Model file for the job. Use its own axes, mm. Give positions to 0.01 mm unless a question says otherwise; leave off trailing zeros. Order: outer loops, then holes, each group sorted by start corner. A loop starts at its lowest first (then second) coordinate and runs counter-clockwise, first axis right, second up. Notation, with made-up numbers: (-39, 56.25) - (-9, 56.25) arc R32 cw to (-9, 86.25) - close; hole circle Ø7 at (59.5, -6.5). An arc over 180 degrees is marked (long way). Return JSON: item names as keys, results as strings. Group by question number.
from build123d import *

# Parameters (mm, degrees)
HEX_2_DEPTH   = 60
BORE_SKETCH_W = 62
BORE_SKETCH_H = 1.5


with BuildPart() as part:
    # Hex Sketch → Hex 2 (new body)
    with BuildSketch(Plane(origin=(0, 0, 0), x_dir=(0, 0, -1), z_dir=(1, 0, 0))):
        Polygon((3.175426481, 0), (1.58771324, 2.75), (-1.58771324, 2.75), (-3.175426481, 0), (-1.58771324, -2.75), (1.58771324, -2.75), align=None)
    extrude(amount=HEX_2_DEPTH)

    # Bore Sketch → Bore (revolve, cut)
    with BuildSketch(Plane.XY, mode=Mode.PRIVATE) as bore_sk:
        with Locations((30, 0.75)):
            Rectangle(BORE_SKETCH_W, BORE_SKETCH_H)
    revolve(bore_sk.sketch.rotate(Axis((-400, 0, 0), (1, 0, 0)), 270), axis=Axis((-400, 0, 0), (1, 0, 0)), mode=Mode.SUBTRACT)


solid = part.part
(1) Drill centre lines: L1, parallel to Y at x = 14, z = 0; L2, parallel to Z at x = 54, y = -0.15; L3, parallel to Y at x = 23, z = -0.75. Where is each one in solid material? Low to high.
(2) Drop a flat-ended pin along its axis: pin 1 Ø1.5 at (x, y) = (27.5, -0.5) entering from +Z. Give the stop position or say it passes through.
(3) Slice it at B-B (y = -0.95). Give the cut face in (x, z).
(4) Slice it at A-A (z = 0). Give the cut face in (x, y).
(5) Slice it at C-C (x = 42). Give the cut face in (y, z), and give its area (3 significant figures).
(6) Slice it at D-D (y = 2.15). Give the cut face in (x, z).
Result set:
{
 "1": {"L1": "y = -2.75 to -1.5, 1.5 to 2.75", "L2": "z = -3.09 to -1.49, 1.49 to 3.09", "L3": "y = -2.75 to -1.3, 1.3 to 2.75"},
 "2": {"pin 1": "stops at z = 3.18"},
 "3": {"outline": "(0, -2.63) - (60, -2.63) - (60, -1.16) - (0, -1.16) - close; (0, 1.16) - (60, 1.16) - (60, 2.63) - (0, 2.63) - close"},
 "4": {"outline": "(0, -2.75) - (60, -2.75) - (60, -1.5) - (0, -1.5) - close; (0, 1.5) - (60, 1.5) - (60, 2.75) - (0, 2.75) - close"},
 "5": {"outline": "(-2.75, -1.59) - (0, -3.18) - (2.75, -1.59) - (2.75, 1.59) - (0, 3.18) - (-2.75, 1.59) - close; hole circle Ø3 at (0, 0)", "area": "19.1 mm²"},
 "6": {"outline": "(0, -1.93) - (60, -1.93) - (60, 1.93) - (0, 1.93) - close"}
}
